The model under review builds one solid part; all positions refer to its coordinate system, in mm. A direction names the side the tool comes from. Give positions to 0.01 mm unless a question says otherwise; leave off trailing zeros. Order: outer loops, then holes, each group sorted by start corner. A loop starts at its lowest first (then second) coordinate and runs counter-clockwise, first axis right, second up. Notation, with made-up numbers: (24, 19.25) - (74, 19.25) arc R18 ccw to (74, 24.25) - close; hole circle Ø7 at (81.5, 74.5). An arc over 180 degrees is marked (long way). Write item = value, one per line. Start each with the question number.
1. Machinability: for faces 1 (the flat face through (-25, 20, 27)), 2 (the flat face through (-139, 15, 29)), 3 (the flat face through (-136, 4, 35)), 4 (the flat face through (-25, 10, 27)), 5 (the flat face through (-250, 20, 27)), which of the approach directions +Z, -Z, +X, -X, +Y, -Y give a long, thin tool a straight path to every point of the face, cutting with its end or side? Answer none if there is none.
2. Mouldability with a two-part tool opening along X and no side actions: class faces 6 (the flat face through (-254, 15, 25)), 7 (the flat face through (-21, 15, 25)), 8 (the flat face through (-250, 15, 21)), 9 (the flat face through (-242, 15, 14)) as pulls with the +X half, pulls with the -X half, needs draft (parallel to the pull), parting line crosses it, or undercut.
3. We need section B-B, the plane y = 27. Give the boundary of the cut face in (x, z), and give its area (3 significant figures).
4. For P1, Ø5, axis at x = -7.5, y = 4.5, coming from the +Z side; P2, Ø2.5, axis at y = 9.4, z = 17.5, coming from the -X side; P3, Ø5.5, axis at x = -24.5, z = 24.5, coming from the -Y side; P4, Ø1.5, axis at y = 10.5, z = 9.5, coming from the +X side, all flat-tipped, find the tip position at first contact; note any pin that passes through.
5. We need section A-A, the plane z = 7. Give the boundary of the cut face in (x, y).
6. We need section C-C, the plane x = -60. Give the boundary of the cut face in (y, z), and give its area (3 significant figures).
7. Wall thickness on probe 1 along X at (y, z) = (11.5, 17.5); probe 2 along Y at (x, z) = (-187.5, 32.1); probe 3 along Z at (x, y) = (-78, 21.25): over which ranges is each line inside the solid? List them lowest first.
from build123d import *

# Parameters (mm, degrees)
SKETCH007_W            = 275
SKETCH007_H            = 30
PAD003_DEPTH           = 36
SKETCH008_W            = 9
SKETCH008_H            = 1
POCKET004_DEPTH        = 275
SKETCH009_R            = 1.5
POCKET005_DEPTH        = 6
LINEARPATTERN001_COUNT = 14
LINEARPATTERN001_PITCH = 20
SKETCH017_W            = 29
SKETCH017_H            = 29
SKETCH017_W_2          = 209
POCKET010_DEPTH        = 30
SKETCH018_R            = 1.5
POCKET011_DEPTH        = 275
SKETCH062_W            = 8
SKETCH062_H            = 8
SKETCH062_R            = 2.2
PAD020_DEPTH           = 5


with BuildPart() as part:
    # Sketch007 → Pad003 (new body)
    with BuildSketch(Plane.XY):
        with Locations((-137.5, 15)):
            Rectangle(SKETCH007_W, SKETCH007_H)
    extrude(amount=PAD003_DEPTH)

    # Sketch008 (on Face2 of Pad003) → Pocket004 (cut)
    with BuildSketch(Plane.YZ):
        with Locations((4.5, 35.5)):
            Rectangle(SKETCH008_W, SKETCH008_H)
    extrude(amount=-POCKET004_DEPTH, mode=Mode.SUBTRACT)

    # Sketch009 (on Face5 of Pocket004) → Pocket005 (cut)
    with BuildSketch(Plane.XY.offset(36)):
        with Locations((-7.5, 4.5)):
            Circle(SKETCH009_R)
    pocket005 = extrude(amount=-POCKET005_DEPTH, mode=Mode.SUBTRACT)

    # LinearPattern001: Pocket005 ×14
    with Locations(*[(-i * LINEARPATTERN001_PITCH, 0, 0) for i in range(1, LINEARPATTERN001_COUNT)]):
        add(pocket005, mode=Mode.SUBTRACT)

    # Sketch017 → Pocket010 (cut)
    with BuildSketch(Plane.XZ):
        with Locations((-14.5, 14.5)):
            Rectangle(SKETCH017_W, SKETCH017_H)
        with Locations((-260.5, 14.5)):
            Rectangle(SKETCH017_W, SKETCH017_H)
        with Locations((-137.5, 14.5)):
            Rectangle(SKETCH017_W_2, SKETCH017_H)
    extrude(amount=-POCKET010_DEPTH, mode=Mode.SUBTRACT)

    # Sketch018 → Pocket011 (cut)
    with BuildSketch(Plane.YZ):
        with Locations((9.4, 17.5)):
            Circle(SKETCH018_R)
        with Locations((19.4, 17.5)):
            Circle(SKETCH018_R)
        with Locations((9.4, 2.5)):
            Circle(SKETCH018_R)
        with Locations((19.4, 2.5)):
            Circle(SKETCH018_R)
    extrude(amount=-POCKET011_DEPTH, mode=Mode.SUBTRACT)

    # Sketch062 → Pad020 (join, symmetric)
    with BuildSketch(Plane.XZ.offset(-15)):
        with Locations((-250, 25)):
            Rectangle(SKETCH062_W, SKETCH062_H)
        with Locations((-250.5, 24.5)):
            Circle(SKETCH062_R, mode=Mode.SUBTRACT)
        with Locations((-25, 25)):
            Rectangle(SKETCH062_W, SKETCH062_H)
        with Locations((-24.5, 24.5)):
            Circle(SKETCH062_R, mode=Mode.SUBTRACT)
    extrude(amount=PAD020_DEPTH, both=True)


solid = part.part
Model answer:
q1.face_1 = -Z, +X, +Y
q1.face_2 = -Z, +Y, -Y
q1.face_3 = +Z, +X, -X, -Y
q1.face_4 = -Z, +X, -Y
q1.face_5 = -Z, -X, +Y
q2.face_6 = pulls with the -X half
q2.face_7 = pulls with the +X half
q2.face_8 = needs draft
q2.face_9 = undercut
q3.outline = (-275, 29) - (-246, 29) - (-246, 0) - (-242, 0) - (-242, 29) - (-33, 29) - (-33, 0) - (-29, 0) - (-29, 29) - (0, 29) - (0, 36) - (-275, 36) - close
q3.area = 2,160 mm2
q4.P1 = 35
q4.P2 = through
q4.P3 = 10
q4.P4 = -29
q5.outline = (-246, 0) - (-242, 0) - (-242, 30) - (-246, 30) - close; (-33, 0) - (-29, 0) - (-29, 30) - (-33, 30) - close
q6.outline = (0, 29) - (30, 29) - (30, 36) - (9, 36) - (9, 35) - (0, 35) - close
q6.area = 201 mm2
q7.probe_1 = -246 to -242, -33 to -29
q7.probe_2 = 0 to 3, 6 to 30
q7.probe_3 = 29 to 36
